from build123d import *

# Parameters (mm, degrees)
PAD_DEPTH       = 25
SKETCH002_R     = 1.85
PAD002_DEPTH    = 15
FILLET_R        = 1
FILLET001_R     = 1
SKETCH004_R     = 2.1
PAD003_DEPTH    = 2
FILLET004_R     = 0.05
FILLET005_R     = 0.4
SKETCH007_W     = 37.33329
SKETCH007_H     = 1
POCKET002_DEPTH = 5
FILLET009_R     = 0.3


with BuildPart() as part:
    # Sketch → Pad (new body)
    with BuildSketch(Plane.XZ):
        with BuildLine():
            Line((0, -25), (0, 25))
            ThreePointArc((0, 25), (-4.774575, 27.95085), (-10, 30))
            Line((-10, -30), (-10, 30))
            ThreePointArc((-10, -30), (-4.774575, -27.95085), (0, -25))
        make_face()
    extrude(amount=PAD_DEPTH)

    # Sketch002 (on Face4 of Pad) → Pad002 (join)
    with BuildSketch(Plane(origin=(-10, 0, 0), x_dir=(0, 0, -1), z_dir=(-1, 0, 0))):
        with Locations((-15, 12.5)):
            Circle(SKETCH002_R)
        with Locations((15, 12.5)):
            Circle(SKETCH002_R)
    extrude(amount=PAD002_DEPTH)

    # Fillet
    fillet_edges = [part.edges().sort_by_distance(p)[0] for p in [
        (-10, -12.5, 30),
        (-10, -25, 0),
        (-10, 0, 0),
        (-10, -12.5, -30),
    ]]
    fillet(fillet_edges, radius=FILLET_R)

    # Fillet001
    fillet001_edges = [part.edges().sort_by_distance(p)[0] for p in [
        (0, 0, 0),
        (0, -25, 0),
    ]]
    fillet(fillet001_edges, radius=FILLET001_R)

    # Sketch004 (on Face16 of Fillet001) → Pad003 (join)
    with BuildSketch(Plane(origin=(-25, 0, 0), x_dir=(0, 0, -1), z_dir=(-1, 0, 0))):
        with Locations((15, 12.5)):
            Circle(SKETCH004_R)
        with Locations((-15, 12.5)):
            Circle(SKETCH004_R)
    extrude(amount=PAD003_DEPTH)

    # Fillet004
    fillet004_edges = [part.edges().sort_by_distance(p)[0] for p in [
        (-25, -12.5, -13.15),
        (-25, -12.5, 16.85),
    ]]
    fillet(fillet004_edges, radius=FILLET004_R)

    # Fillet005
    fillet005_edges = [part.edges().sort_by_distance(p)[0] for p in [
        (-27, -12.5, -12.9),
        (-27, -12.5, 17.1),
    ]]
    fillet(fillet005_edges, radius=FILLET005_R)

    # Sketch007 (on Face24 of Fillet005) → Pocket002 (cut)
    with BuildSketch(Plane(origin=(-27, 0, 0), x_dir=(0, 0, -1), z_dir=(-1, 0, 0))):
        with Locations((0.43578, 12.5)):
            Rectangle(SKETCH007_W, SKETCH007_H)
    extrude(amount=-POCKET002_DEPTH, mode=Mode.SUBTRACT)

    # Fillet009
    fillet009_edges = [part.edges().sort_by_distance(p)[0] for p in [
        (-22, -12, 15),
        (-22, -13, 15),
        (-22, -13, -15),
        (-22, -12, -15),
    ]]
    fillet(fillet009_edges, radius=FILLET009_R)


solid = part.part
The model under review builds one solid part; all positions refer to its coordinate system, in mm. A direction names the side the tool comes from. Coordinates: 2 decimals unless noted, no trailing zeros. Loops run counter-clockwise (first coordinate to the right, second up) from the corner with the lowest first, then second, coordinate; pieces in that order, holes last. Notation, with made-up numbers: (-37.75, 45) -> (-29.75, 45) arc R17 cw to (-29.75, 64) -> close; hole circle Ø8 at (15, 24.5). An arc over 180 degrees is marked (long way). Use a Markdown table: item, result. Add a question column.
1. Add section B-B on x = -23.25. Write out the cut boundary in (y, z).
2. Add section D-D on z = 15. Write out the cut boundary in (x, y), plus the area to 3 significant figures.
3. Add section C-C on y = -4.75. Write out the cut boundary in (x, z).
4. Draft analysis for pull direction X (two halves, no side actions). For faces 5 (the face through (-9.571, -12.675, -29.456)), 6 (the face through (-17.37, -11.79, -16.71)), 7 (the face through (-5, -25, 0)), 8 (the face through (-27, -13.5, 15)), state which applies: pulls with the +X half, pulls with the -X half, needs draft (parallel to the pull), parting line crosses it, or undercut.
5. Add section A-A on z = -23. Write out the cut boundary in (x, y).
6. To check wall thickness, follow line 1 (X direction, y = -21.75, z = 1); line 2 (Y direction, x = -25.5, z = -16.5); line 3 (Z direction, x = -4, y = -10.25). State the ranges of each line that lie inside material, in increasing order.
7. Clearance check with flat-ended pins moving along their axes: pin 1 Ø2 at (x, z) = (-25, 15.5) entering from -Y; pin 2 Ø2 at (x, z) = (-24.5, -14.5) entering from +Y; pin 3 Ø1.5 at (x, z) = (-24, 13.5) entering from +Y. State where each tip first meets the part, or that it passes through.
8. Machinability: for faces 1 (the face through (-25.8, -10.4, -15)), 2 (the face through (-25.8, -14.6, -15)), 3 (the face through (-17.37, -11.79, 13.29)), 4 (the face through (-25, -12, -15)), which of the approach directions +Z, -Z, +X, -X, +Y, -Y give a long, thin tool a straight path to every point of the face, cutting with its end or side? Answer none if there is none.
Returned:
| question | item | result |
|---|---|---|
| 1 | outline | (-13, -16.78) -> (-13, -13.22) arc R1.85 ccw to start; (-13, 13.22) -> (-13, 16.78) arc R1.85 ccw to start; (-12, -16.78) arc R1.85 ccw to (-12, -13.22) -> close; (-12, 13.22) arc R1.85 ccw to (-12, 16.78) -> close |
| 2 | outline | (-27, -14.2) arc R0.4 ccw to (-26.6, -14.6) -> (-25, -14.6) -> (-25, -14.4) arc R0.05 cw to (-24.95, -14.35) -> (-10, -14.35) -> (-10, -24) arc R1 ccw to (-9, -25) -> (-1, -25) arc R1 ccw to (0, -24) -> (0, -1) arc R1 ccw to (-1, 0) -> (-9, 0) arc R1 ccw to (-10, -1) -> (-10, -10.65) -> (-24.95, -10.65) arc R0.05 cw to (-25, -10.6) -> (-25, -10.4) -> (-26.6, -10.4) arc R0.4 ccw to (-27, -10.8) -> (-27, -12) -> (-22.3, -12) arc R0.3 cw to (-22, -12.3) -> (-22, -12.7) arc R0.3 cw to (-22.3, -13) -> (-27, -13) -> close |
| 2 | area | 308 mm² |
| 3 | outline | (-10, -28.64) arc R1 ccw to (-8.68, -29.58) arc R31.25 ccw to (0, -25) -> (0, 25) arc R31.25 ccw to (-8.68, 29.58) arc R1 ccw to (-10, 28.64) -> close |
| 4 | face 5 | parting line crosses it |
| 4 | face 6 | undercut |
| 4 | face 7 | needs draft |
| 4 | face 8 | pulls with the -X half |
| 5 | outline | (-10, -24) arc R1 ccw to (-9, -25) -> (-1, -25) arc R1 ccw to (0, -24) -> (0, -1) arc R1 ccw to (-1, 0) -> (-9, 0) arc R1 ccw to (-10, -1) -> close |
| 6 | line 1 | x = -10 to 0 |
| 6 | line 2 | y = -13.97 to -13, -12 to -11.03 |
| 6 | line 3 | z = -27.55 to 27.55 |
| 7 | pin 1 | stops at y = -14.6 |
| 7 | pin 2 | stops at y = -10.4 |
| 7 | pin 3 | stops at y = -10.81 |
| 8 | face 1 | -X, +Y |
| 8 | face 2 | -X, -Y |
| 8 | face 3 | none |
| 8 | face 4 | +Z, -Z, -X |
